The model under review builds one solid part; all positions refer to its coordinate system, in mm. A direction names the side the tool comes from. Round coordinates to 2 decimals unless told otherwise and drop trailing zeros. Loops run counter-clockwise (first coordinate to the right, second up) from the corner with the lowest first, then second, coordinate; pieces in that order, holes last. Notation, with made-up numbers: M 49.5,76.5 L 90.5,76.5 A10 ccw 90.5,85.5 Z; hole C -6.5,-16 d9. An arc over 180 degrees is marked long. Return JSON: item names as keys, results as strings. Group by question number.
Q1. Consider section C-C (x = -182). State the section outline as (y, z) points.
Q2. For faces 1 (the face through (355.6, -45, 235)), 2 (the face through (-149, -82.55, 186)), 3 (the face through (329.84, -46.51, 225.65)), list the 3-axis set-ups (+Z, -Z, +X, -X, +Y, -Y) from which the entire face can be reached by the end or side of a thin tool; tool diameter is ignored.
Q3. Consider section B-B (y = -21). State the section outline as (x, z) points, and give its area (3 significant figures).
Q4. Consider section A-A (z = 0). State the section outline as (x, y) points.
Q5. Consider section D-D (z = -210). State the section outline as (x, y) points.
Q6. Clearance check with flat-ended pins moving along their axes: pin 1 Ø1.5 at (x, y) = (-18, -27.5) entering from +Z; pin 2 Ø3 at (y, z) = (-87, 140.5) entering from +X. State where each tip first meets the part, or that it passes through.
Q7. Draft analysis for pull direction Z (two halves, no side actions). For faces 4 (the face through (-71, -6.35, 70)), 5 (the face through (-2.572, -3.219, -76.157)), 6 (the face through (-4, -44, -254)), state which applies: pulls with the +Z half, pulls with the -Z half, needs draft (parallel to the pull), parting line crosses it, or undercut.
Q8. To check wall thickness, follow line 1 along X through (y, z) = (-3, 0); line 2 along X through (y, z) = (-50.5, -172.5); line 3 along Y through (x, z) = (167, 219). State the ranges of each line that lie inside material, in increasing order.
from build123d import *

# Parameters (mm, degrees)
F0_W      = 609.6
F0_H      = 508
F1_DEPTH  = 88.9
F2_W      = 596.9
F2_H      = 82.55
F3_DEPTH  = 482.6
F4_R      = 9.525
F5_DEPTH  = 50.8
F7_DEPTH  = 82.55
F8_W      = 152.4
F8_H      = 304.8
F9_DEPTH  = 82.55
F11_DEPTH = 6.35
F12_R     = 76.2
F13_DEPTH = 25.4
F14_W     = 101.6
F14_H     = 177.8
F15_DEPTH = 25.4
F16_W     = 101.6
F16_H     = 199.39
F17_DEPTH = 25.4


with BuildPart() as f1:
    # F0 (on Front) → F1 (new body)
    with BuildSketch(Plane.XZ):
        Rectangle(F0_W, F0_H)
    extrude(amount=F1_DEPTH)

    # F2 (on face) → F3 (cut)
    with BuildSketch(Plane.XY.offset(254)):
        with Locations((0, -47.625)):
            Rectangle(F2_W, F2_H)
    extrude(amount=-F3_DEPTH, mode=Mode.SUBTRACT)

    # F4 (on face) → F5 (join)
    with BuildSketch(Plane.YZ.offset(304.8)):
        with Locations((-44.45, 234.95)):
            Circle(F4_R)
    extrude(amount=F5_DEPTH)

    # F6 (on face) → F7 (join, through all)
    with BuildSketch(Plane.XZ.offset(88.9)):
        Polygon((-298.45, 254), (-298.45, 76.2), (-146.05, 76.2), align=None)
        Polygon((298.45, 254), (146.05, 76.2), (298.45, 76.2), align=None)
    extrude(amount=-F7_DEPTH)

    # F8 (on face) → F9 (join, through all)
    with BuildSketch(Plane.XZ.offset(88.9)):
        with Locations((-222.25, -76.2)):
            Rectangle(F8_W, F8_H)
        with Locations((222.25, -76.2)):
            Rectangle(F8_W, F8_H)
    extrude(amount=-F9_DEPTH)

    # F10 (on face) → F11 (join)
    with BuildSketch(Plane.XZ.offset(88.9)):
        Polygon((298.45, 254), (-298.45, 254), (-146.05, 76.2), (146.05, 76.2), align=None)
    extrude(amount=-F11_DEPTH)

    # F12 (on face) → F13 (cut)
    with BuildSketch(Plane.XZ.offset(6.35)):
        Circle(F12_R)
    extrude(amount=-F13_DEPTH, mode=Mode.SUBTRACT)

    # F14 (on face) → F15 (cut)
    with BuildSketch(Plane.XZ.offset(88.9)):
        with Locations((0, 165.1)):
            Rectangle(F14_W, F14_H)
    extrude(amount=-F15_DEPTH, mode=Mode.SUBTRACT)

    # F16 (on face) → F17 (cut)
    with BuildSketch(Plane.XZ):
        with Locations((0, 154.305)):
            Rectangle(F16_W, F16_H)
    extrude(amount=F17_DEPTH, mode=Mode.SUBTRACT)


solid = f1.part
Values:
{
 "1": {"outline": "M -88.9,-254 L 0,-254 L 0,254 L -6.35,254 L -6.35,118.14 L -82.55,118.14 L -82.55,254 L -88.9,254 Z"},
 "2": {"face 1": "+Z, -Z, +X, +Y, -Y", "face 2": "+Z", "face 3": "+X"},
 "3": {"outline": "M -304.8,-254 L 304.8,-254 L 304.8,254 L 298.45,254 L 146.05,76.2 L 146.05,-228.6 L -146.05,-228.6 L -146.05,76.2 L -298.45,254 L -304.8,254 Z", "area": "142,000 mm2"},
 "4": {"outline": "M -304.8,-88.9 L -146.05,-88.9 L -146.05,-6.35 L -76.2,-6.35 L -76.2,0 L -304.8,0 Z; M 76.2,-6.35 L 146.05,-6.35 L 146.05,-88.9 L 304.8,-88.9 L 304.8,0 L 76.2,0 Z"},
 "5": {"outline": "M -304.8,-88.9 L -146.05,-88.9 L -146.05,-6.35 L 146.05,-6.35 L 146.05,-88.9 L 304.8,-88.9 L 304.8,0 L -304.8,0 Z"},
 "6": {"pin 1": "stops at z = -228.6", "pin 2": "stops at x = 304.8"},
 "7": {"face 4": "needs draft", "face 5": "undercut", "face 6": "pulls with the -Z half"},
 "8": {"line 1": "x = -304.8 to -76.2, 76.2 to 304.8", "line 2": "x = -304.8 to -146.05, 146.05 to 304.8", "line 3": "y = -88.9 to -82.55, -6.35 to 0"}
}
